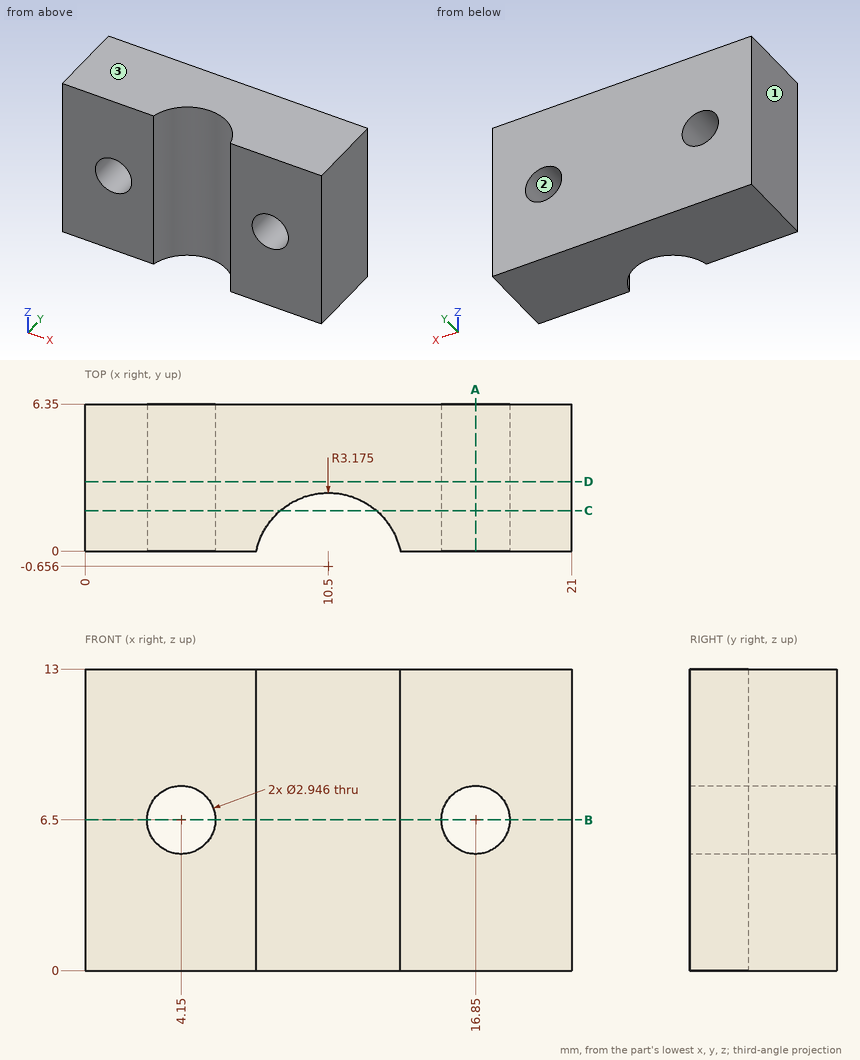
Print and shaded views of the part. All mm, measured from the part's lowest x, y and z. Coordinates: 2 decimals unless noted, no trailing zeros. Write each loop counter-clockwise with the first axis right and the second up, starting at its lowest first coordinate (ties: lowest second). Pieces come first, ordered by that corner, then holes. Notation, with made-up numbers: (85, -36.5) - (124, -36.5) arc R17 cw to (124, -6.5) - close; hole circle Ø6 at (-10, 42). An arc over 180 degrees is marked (long way). One line per question, with ' | ' between items. Start each with the question number.
Q1. Cut at D-D, the plane y = 3. List the corners of the cut face in (x, z), then the cut area to 3 significant figures.
Q2. Cut at C-C, the plane y = 1.75. List the corners of the cut face in (x, z).
Q3. Pin check, flat tips, straight feed: pin 1 (1.8 mm diameter, centred on x = 16.85, z = 6.5, fed in from +Y); pin 2 (6 mm diameter, centred on x = 9.5, z = 10.5, fed in from -Y). Stop position of each tip, or through.
Q4. Drill centre lines: line 1 (X direction, y = 4.5, z = 6.5); line 2 (X direction, y = 6, z = 7) (1 decimal); line 3 (X direction, y = 1.5, z = 6.5) (1 decimal). Where is each one in solid material? Low to high. Write a range as [from, to].
Q5. Cut at A-A, the plane x = 16.85. List the corners of the cut face in (y, z).
Q6. Pull direction X, two halves, no side cores. Call the marked faces 1, 2 and 3: pulls with the +X half, pulls with the -X half, needs draft (parallel to the pull), parting line crosses it, or undercut.
Q7. Cut at B-B, the plane z = 6.5. Give the number of separate pieces and of enclosed holes in the cut face.
Answer below:
1) outline: (0, 0) - (21, 0) - (21, 13) - (0, 13) - close; hole circle Ø2.95 at (4.15, 6.5); hole circle Ø2.95 at (16.85, 6.5) | area: 259 mm^2
2) outline: (0, 0) - (8.43, 0) - (8.43, 13) - (0, 13) - close; (12.57, 0) - (21, 0) - (21, 13) - (12.57, 13) - close; hole circle Ø2.95 at (4.15, 6.5); hole circle Ø2.95 at (16.85, 6.5)
3) pin 1: through | pin 2: y = 0
4) line 1: [0, 2.68], [5.62, 15.38], [18.32, 21] | line 2: [0, 2.8], [5.5, 15.5], [18.2, 21] | line 3: [0, 2.7], [5.6, 8.2], [12.8, 15.4], [18.3, 21]
5) outline: (0, 0) - (6.35, 0) - (6.35, 5.03) - (0, 5.03) - close; (0, 7.97) - (6.35, 7.97) - (6.35, 13) - (0, 13) - close
6) face 1: pulls with the -X half | face 2: undercut | face 3: needs draft
7) separate pieces: 3 | enclosed holes: 0
